from build123d import *

# Parameters (mm, degrees)
F2_W     = 10
F2_H     = 40
F3_DEPTH = 40.001
F4_D     = 4.5


with BuildPart() as f1:
    # F0 (on Front) → F1 (revolve)
    with BuildSketch(Plane.XZ):
        Polygon((0, 20), (0, 6), (40, 6), (40, 12), (10, 12), (10, 20), align=None)
    revolve(axis=Axis((24.2165401578, 0, 0), (1, 0, 0)))

    # F2 (on face) → F3 (cut, through all)
    with BuildSketch(Plane(origin=(0, 0, 0), x_dir=(0, -1, 0), z_dir=(-1, 0, 0))):
        with Locations((-20, 0)):
            Rectangle(F2_W, F2_H)
        with Locations((20, 0)):
            Rectangle(F2_W, F2_H)
    extrude(amount=-F3_DEPTH, mode=Mode.SUBTRACT)

    # F4 (through all)
    with Locations(Plane(origin=(0, 0, 0), x_dir=(0, -1, 0), z_dir=(-1, 0, 0))):
        with Locations((-11.313708499, 11.313708499), (11.313708499, 11.313708499), (11.313708499, -11.313708499), (-11.313708499, -11.313708499), (0, 16), (0, -16)):
            Hole(F4_D / 2)


solid = f1.part
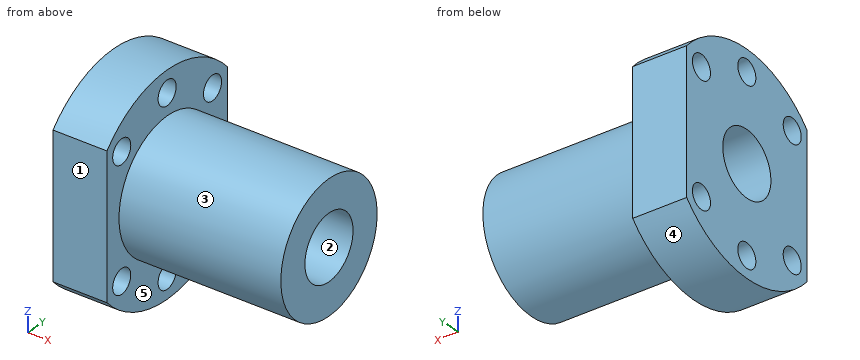
Work out the finished part from the listing and answer in its coordinate system (mm). Face numbers are marked on the shaded views. A direction names the side the tool comes from. Coordinates: 2 decimals unless noted, no trailing zeros. Order: outer loops, then holes, each group sorted by start corner. A loop starts at its lowest first (then second) coordinate and runs counter-clockwise, first axis right, second up. Notation, with made-up numbers: (73.25, 40) - (112.25, 40) arc R17 cw to (112.25, 62) - close; hole circle Ø9 at (0.25, -40). An arc over 180 degrees is marked (long way). Put each result on its own line as item: value. Start each with the question number.
1) Find section C-C (z = -16). Give the vertices of the cut face in (x, y), plus the area to 3 significant figures.
2) Find section A-A (z = 0). Give the vertices of the cut face in (x, y), plus the area to 3 significant figures.
3) For a pull along Z with two mould halves and no side action, classify the marked faces 1, 2 and 3 as released by +Z, released by -Z, zero draft, split by the parting line, or undercut.
4) Find the intervals of material crossed by line 1 (X direction, y = 2, z = 18); line 2 (Z direction, x = 18, y = 0); line 3 (Y direction, x = 20, z = -5.5), in increasing order. Write a range as from..to.
5) For the marked faces 4 and 5, determine the directions among +Z, -Z, +X, -X, +Y, -Y from which every point of the face is accessible in a straight line to the end or side of a thin tool.
6) Find section D-D (y = -4.5). Give the vertices of the cut face in (x, z), plus the area to 3 significant figures.
7) Find section B-B (y = 10). Give the vertices of the cut face in (x, z), plus the area to 3 significant figures.
8) Flat-ended cylindrical pins translate along their axes: pin 1 (1 mm diameter, centred on x = 5.5, y = 11, fed in from +Z); pin 2 (4 mm diameter, centred on y = -11.31, z = -11.31, fed in from +X); pin 3 (5 mm diameter, centred on x = 23.5, y = 3.5, fed in from +Z); pin 4 (1.5 mm diameter, centred on x = 14.5, y = 7.5, fed in from +Z). Find the tip coordinate at first contact, or state that the pin passes through.
Results list:
1. outline: (0, -12) - (10, -12) - (10, -2.25) - (0, -2.25) - close; (0, 2.25) - (10, 2.25) - (10, 12) - (0, 12) - close
1. area: 195 mm^2
2. outline: (0, -15) - (10, -15) - (10, -12) - (40, -12) - (40, -6) - (0, -6) - close; (0, 6) - (40, 6) - (40, 12) - (10, 12) - (10, 15) - (0, 15) - close
2. area: 540 mm^2
3. face 1: zero draft
3. face 2: undercut
3. face 3: split by the parting line
4. line 1: x = 0..10
4. line 2: z = -12..-6, 6..12
4. line 3: y = -10.67..-2.4, 2.4..10.67
5. face 4: -Z, +X, -X
5. face 5: +X
6. outline: (0, -19.49) - (10, -19.49) - (10, -11.12) - (40, -11.12) - (40, -3.97) - (0, -3.97) - close; (0, 3.97) - (40, 3.97) - (40, 11.12) - (10, 11.12) - (10, 19.49) - (0, 19.49) - close
6. area: 740 mm^2
7. outline: (0, -17.32) - (10, -17.32) - (10, -13.14) - (0, -13.14) - close; (0, -9.49) - (10, -9.49) - (10, -6.63) - (40, -6.63) - (40, 6.63) - (10, 6.63) - (10, 9.49) - (0, 9.49) - close; (0, 13.14) - (10, 13.14) - (10, 17.32) - (0, 17.32) - close
7. area: 671 mm^2
8. pin 1: stops at z = 17.02
8. pin 2: passes through
8. pin 3: stops at z = 11.96
8. pin 4: stops at z = 9.92
